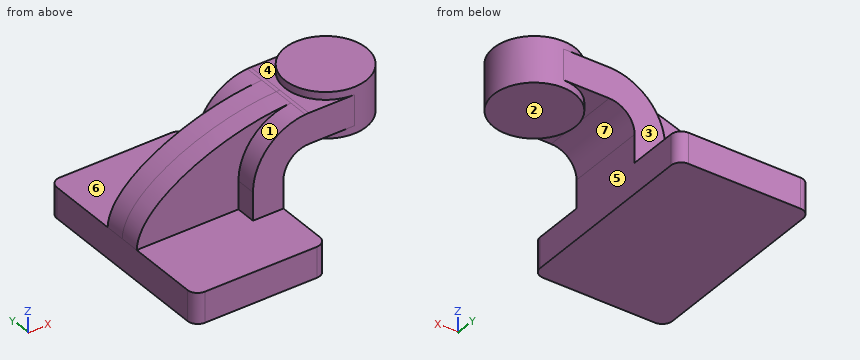
```python
from build123d import *

# Parameters (mm, degrees)
F1_DEPTH = 63.5
F0_W     = 25.4
F0_H     = 19.05
F2_DEPTH = 25.4
F3_DEPTH = 12.7
F5_R     = 6.35


with BuildPart() as f1:
    # F0 (on Front) → F1 (new body, symmetric)
    with BuildSketch(Plane.XZ):
        Polygon((41.275, -9.525), (41.275, 9.525), (22.225, 9.525), (-41.275, 9.525), (-41.275, -9.525), align=None)
    extrude(amount=F1_DEPTH, both=True)

    # F0 (on Front) → F2 (join, symmetric)
    with BuildSketch(Plane.XZ):
        with BuildLine():
            Line((22.225, 9.525), (41.275, 9.525))
            Line((41.275, 9.525), (41.275, 27.0002))
            ThreePointArc((41.275, 27.0002), (45.92468, 38.22552), (57.15, 42.8752))
            Line((57.15, 42.8752), (60.325, 42.8752))
            Line((60.325, 42.8752), (60.325, 61.9252))
            Line((60.325, 61.9252), (57.15, 61.9252))
            add(Edge.make_bspline(
                [(54.968883, 61.857026), (55.698999, 61.886176), (56.426142, 61.908931), (57.15, 61.9252)],
                knots=[109.624995, 109.624995, 109.624995, 109.624995, 111.504536, 111.504536, 111.504536, 111.504536], degree=3))
            ThreePointArc((54.968883, 61.857026), (31.694832, 50.912332), (22.225, 27.0002))
            Line((22.225, 27.0002), (22.225, 9.525))
        make_face()
        with Locations((73.025, 52.4002)):
            Rectangle(F0_W, F0_H)
    extrude(amount=F2_DEPTH, both=True)

    # F0 (on Front) → F3 (join, symmetric)
    with BuildSketch(Plane.XZ):
        with BuildLine():
            Line((-41.275, 9.525), (22.225, 9.525))
            Line((22.225, 9.525), (22.225, 27.0002))
            ThreePointArc((22.225, 27.0002), (31.694832, 50.912332), (54.968883, 61.857026))
            add(Edge.make_bspline(
                [(-41.275, 9.525), (-40.314914, 36.701423), (12.384545, 60.156845), (54.968883, 61.857026)],
                knots=[0, 0, 0, 0, 109.624995, 109.624995, 109.624995, 109.624995], degree=3))
        make_face()
    extrude(amount=F3_DEPTH, both=True)

    # F0 (on Front) → F4 (revolve)
    with BuildSketch(Plane.XZ):
        Polygon((85.725, 61.9252), (85.725, 42.8752), (85.725, 38.1), (111.125, 38.1), (111.125, 66.675), (85.725, 66.675), align=None)
    revolve(axis=Axis((85.725, 0, 52.3875), (0, 0, 1)))

    # F5
    f5_edges = [f1.edges().sort_by_distance(p)[0] for p in [
        (41.275, -63.5, 0),
        (-41.275, -63.5, 0),
        (-41.275, 63.5, 0),
        (41.275, 63.5, 0),
    ]]
    fillet(f5_edges, radius=F5_R)


solid = f1.part
```
Input: part model. Units: mm. Frame: model coordinates. Face numbers are marked on the shaded views. A direction names the side the tool comes from. Coordinates: 2 decimals unless noted, no trailing zeros. Write each loop counter-clockwise with the first axis right and the second up, starting at its lowest first coordinate (ties: lowest second). Pieces come first, ordered by that corner, then holes.
1) Material intervals for line 1 along Y through (x, z) = (63.5, 56.5); line 2 along Z through (x, y) = (102.5, 12.5) (3 decimals); line 3 along Z through (x, y) = (36.5, -32.5) (3 decimals), sorted ascending.
2) Section B-B on y = 32. Output: boundary loops of the cut face in (x, z) (3 decimals).
3) Section C-C on x = 69. Output: boundary loops of the cut face in (y, z) (3 decimals), and give its area (3 significant figures).
4) Section A-A on z = 5. Output: boundary loops of the cut face in (x, y) (3 decimals).
5) Mould query, pull axis X, two halves, no side actions, for the marked faces 5, 6 and 7. Classes: pulls with the +X half, pulls with the -X half, needs draft (parallel to the pull), parting line crosses it, or undercut.
6) Set-up query: the marked faces 1, 2, 3 and 4. Return all of +Z, -Z, +X, -X, +Y, -Y with unobstructed straight access to the full face (end or side cutting, diameter ignored); none if empty.
7) Pin query (flat end, axial travel): pin 1 Ø2 at (x, y) = (3, -33) entering from +Z (3 decimals); pin 2 Ø8.5 at (x, y) = (72.5, 4) entering from -Z; pin 3 Ø12 at (x, z) = (19, 49) entering from +Y. Return the tip coordinate at first contact, or that it passes through.
Check result:
1. line 1: y = -25.4 to 25.4
1. line 2: z = 38.1 to 66.675
1. line 3: z = -9.525 to 9.525
2. outline: (-41.275, -9.525) - (41.275, -9.525) - (41.275, 9.525) - (-41.275, 9.525) - close
3. outline: (-25.4, 42.875) - (-19.116, 42.875) - (-19.116, 38.1) - (19.116, 38.1) - (19.116, 42.875) - (25.4, 42.875) - (25.4, 61.925) - (19.116, 61.925) - (19.116, 66.675) - (-19.116, 66.675) - (-19.116, 61.925) - (-25.4, 61.925) - close
3. area: 1,330 mm2
4. outline: (-41.275, -57.15) arc R6.35 ccw to (-34.925, -63.5) - (34.925, -63.5) arc R6.35 ccw to (41.275, -57.15) - (41.275, 57.15) arc R6.35 ccw to (34.925, 63.5) - (-34.925, 63.5) arc R6.35 ccw to (-41.275, 57.15) - close
5. face 5: pulls with the +X half
5. face 6: needs draft
5. face 7: undercut
6. face 1: +Z, -X, -Y
6. face 2: -Z, +X, +Y, -Y
6. face 3: +Z, +X, -X, +Y
6. face 4: +Z, -X
7. pin 1: stops at z = 9.525
7. pin 2: stops at z = 38.1
7. pin 3: stops at y = 12.7
